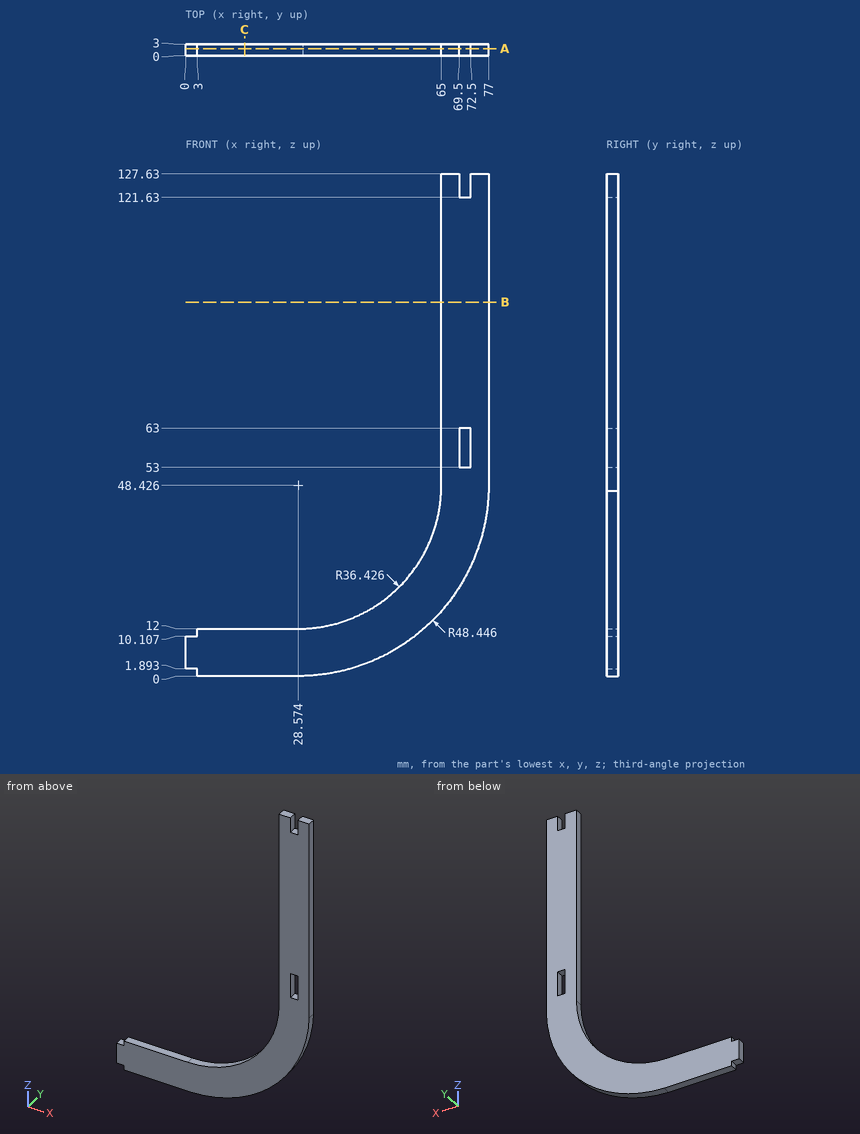
Geometry check sheet. Reference: drawing and pictorial views, mm from the part's lowest x, y, z. Give positions to 0.01 mm unless a question says otherwise; leave off trailing zeros. Write each loop counter-clockwise with the first axis right and the second up, starting at its lowest first coordinate (ties: lowest second). Pieces come first, ordered by that corner, then holes.
Item 1: Cross-section at C-C (x = 15). Enter the section's corners in (y, z).
Item 2: Cross-section at B-B (z = 95). Enter the section's corners in (x, y), and give its area (3 significant figures).
Item 3: Gauge pin test, flat ends, axial feed: pin 1 (1.5 mm diameter, centred on x = 1.5, y = 2, fed in from +Z); pin 2 (4 mm diameter, centred on x = 61.5, z = 36, fed in from -Y); pin 3 (0.9 mm diameter, centred on x = 1.5, y = 1.5, fed in from -Z); pin 4 (1.5 mm diameter, centred on y = 1, z = 80.5, fed in from -X). Record the tip position at first contact, or that the pin passes through.
Item 4: Scan lines: L1, parallel to X at y = 1.45, z = 122; L2, parallel to X at y = 1.65, z = 96; L3, parallel to Z at x = 5, y = 1.7. Record each from-to range of solid material in increasing order.
Item 5: Cross-section at A-A (y = 1.85). Enter the section's corners in (x, z), and give its area (4 significant figures).
Report:
1. outline: (0, 0) - (3, 0) - (3, 12) - (0, 12) - close
2. outline: (65, 0) - (77, 0) - (77, 3) - (65, 3) - close
2. area: 36.0 mm2
3. pin 1: stops at z = 10.11
3. pin 2: stops at y = 0
3. pin 3: stops at z = 1.89
3. pin 4: stops at x = 65
4. L1: x = 65 to 69.5, 72.5 to 77
4. L2: x = 65 to 77
4. L3: z = 0 to 12
5. outline: (0, 1.89) - (3, 1.89) - (3, 0) - (29.95, 0) arc R48.45 ccw to (77, 47.05) - (77, 127.63) - (72.5, 127.63) - (72.5, 121.63) - (69.5, 121.63) - (69.5, 127.63) - (65, 127.63) - (65, 48.43) arc R36.43 cw to (28.57, 12) - (3, 12) - (3, 10.11) - (0, 10.11) - close; hole (69.5, 53) - (72.5, 53) - (72.5, 63) - (69.5, 63) - close
5. area: 2,035 mm2
